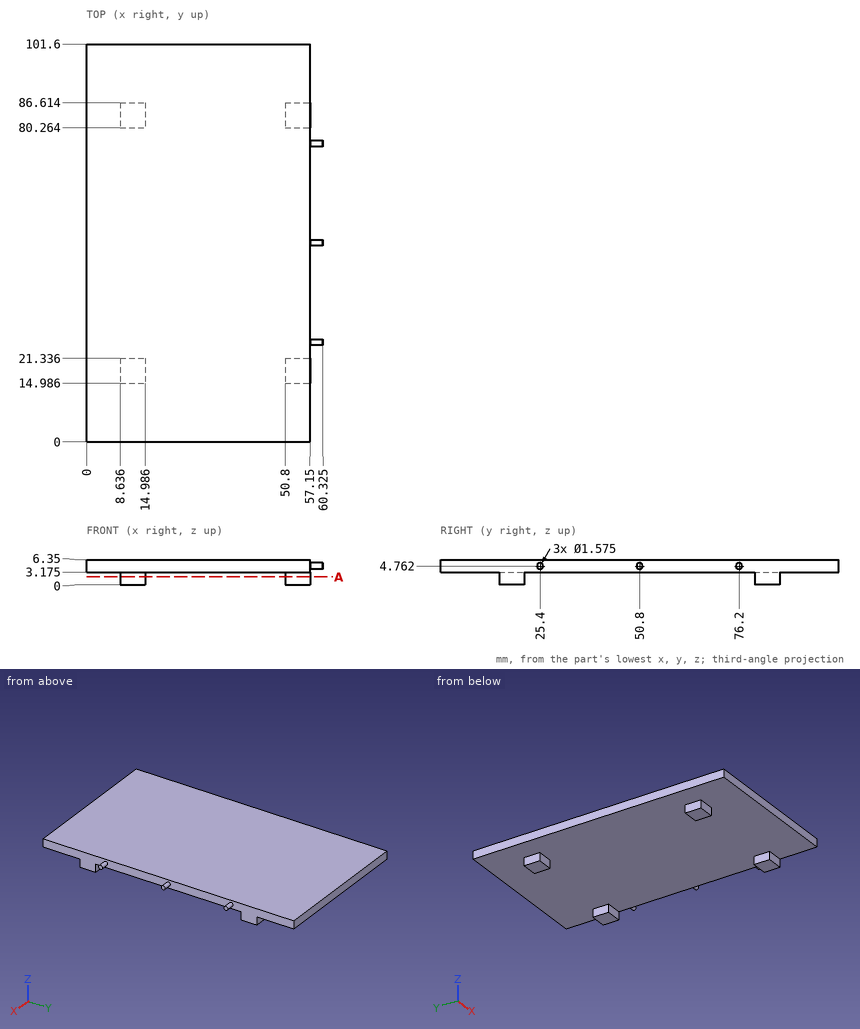
Can you work these out from the drawing? Everything is in mm from the part's minimum corner. Give positions to 0.01 mm unless a question says otherwise; leave off trailing zeros.
1. Suppose I cut it at A-A (z = 2). Give the number of separate pieces and of enclosed holes in the cut face, plus the area to 3 significant figures.
2. I need wall thicknesses on L1, parallel to Y at x = 52, z = 2.5 (1 decimal); L2, parallel to X at y = 83, z = 4.5. Which ranges of each line are inside material? Lowest first, please.
3. Will these pins go through, and if not, where does the flat tip stop? P1, Ø2, axis at x = 47.5, z = 2.5, coming from the +Y side; P2, Ø3.5, axis at y = 82.5, z = 1.5, coming from the +X side; P3, Ø1.6, axis at x = 11.5, z = 1, coming from the -Y side; P4, Ø12, axis at x = 48.5, y = 31.5, coming from the -Z side (1 decimal).
Solved:
1. separate pieces: 4
1. enclosed holes: 0
1. area: 161 mm2
2. L1: y = 15 to 21.3, 80.3 to 86.6
2. L2: x = 0 to 57.15
3. P1: stops at y = 101.6
3. P2: stops at x = 57.15
3. P3: stops at y = 14.99
3. P4: stops at z = 3.2
